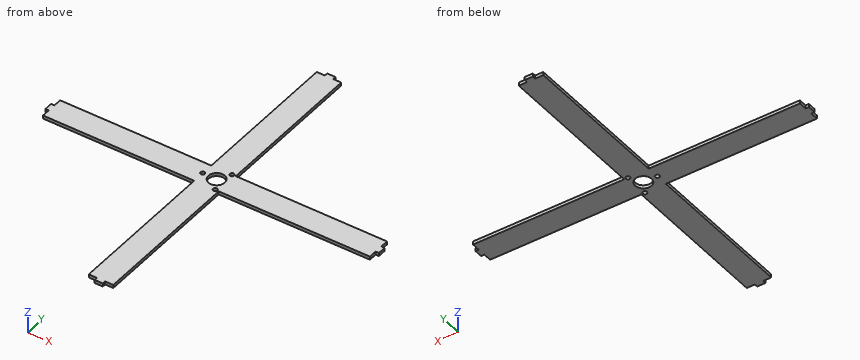
from build123d import *

# Parameters (mm, degrees)
BOSS_EXTRUDE1_DEPTH = 4
CAVITY1_OUTLINE_R   = 2.6
CAVITY1_OUTLINE_R_2 = 10
CAVITY1_DEPTH       = 4


# Read off the part's stored shape, not the designer's step: Cavity1
with BuildPart() as part:
    # Sketch1 → Boss-Extrude1 (new body)
    with BuildSketch(Plane.XY):
        Polygon((363.586470787, 3.889663418), (367.586470787, 3.889663418), (367.586470787, 13.889663418), (363.586470787, 13.889663418), (363.586470787, 23.889663418), (178.577070849, 23.889663418), (178.577070849, 208.900229456), (168.577070849, 208.900229456), (168.577070849, 212.900229456), (158.577070849, 212.900229456), (158.577070849, 208.900229456), (148.577070849, 208.900229456), (148.577070849, 23.889663418), (-36.413529213, 23.889663418), (-36.413529213, 13.889663418), (-40.413529213, 13.889663418), (-40.413529213, 3.889663418), (-36.413529213, 3.889663418), (-36.413529213, -6.110336582), (148.577070849, -6.110336582), (148.577070849, -191.099770544), (158.577070849, -191.099770544), (158.577070849, -195.099770544), (168.577070849, -195.099770544), (168.577070849, -191.099770544), (178.577070849, -191.099770544), (178.577070849, -6.110336582), (363.586470787, -6.110336582), align=None)
    extrude(amount=BOSS_EXTRUDE1_DEPTH)

    # Cavity1 outline → Cavity1 (cut)
    with BuildSketch(Plane.XY):
        with Locations((174.136470787, 23.709263861)):
            Circle(CAVITY1_OUTLINE_R)
        with Locations((174.136470787, -5.908804949)):
            Circle(CAVITY1_OUTLINE_R)
        with Locations((148.486470787, 8.900229456)):
            Circle(CAVITY1_OUTLINE_R)
        with Locations((165.586470787, 8.900229456)):
            Circle(CAVITY1_OUTLINE_R_2)
    extrude(amount=CAVITY1_DEPTH, mode=Mode.SUBTRACT)


solid = part.part
CAD build for the part. Positions are in the model's coordinates, mm. Round coordinates to 2 decimals unless told otherwise and drop trailing zeros. Write each loop counter-clockwise with the first axis right and the second up, starting at its lowest first coordinate (ties: lowest second). Pieces come first, ordered by that corner, then holes. Notation, with made-up numbers: M -34,-34.5 L 10,-34.5 A34 ccw 10,0.5 Z; hole C 64.5,-11.75 d2. An arc over 180 degrees is marked long. Use a Markdown table: item, result. Add a question column.
1. Flat gauge pins, fed straight in: P1, Ø4.5, axis at x = 174.14, y = 23.71, coming from the -Z side; P2, Ø1, axis at y = -5.5, z = 2, coming from the +X side; P3, Ø1, axis at x = 13.5, z = 3, coming from the +Y side; P4, Ø7, axis at x = 148.49, y = 8.9, coming from the +Z side. Where does each tip first touch, or does it go through?
2. Slice it at B-B on x = 185. Give the cut face in (y, z).
3. Slice it at A-A on z = 2.15. Give the number of separate pieces and of enclosed holes in the cut face, then the cut area to 3 significant figures.
4. Drill centre lines: probe 1 along Y at (x, z) = (208, 1.9); probe 2 along Y at (x, z) = (162, 0.4); probe 3 along X at (y, z) = (157, 2.2). Where is each one in solid material? Low to high.
5. Slice it at C-C on y = 155. Give the cut face in (x, z), then the cut area to 3 significant figures.
Reply:
| question | item | result |
|---|---|---|
| 1 | P1 | passes through |
| 1 | P2 | stops at x = 363.59 |
| 1 | P3 | stops at y = 23.89 |
| 1 | P4 | stops at z = 4 |
| 2 | outline | M -6.11,0 L 23.89,0 L 23.89,4 L -6.11,4 Z |
| 3 | separate pieces | 1 |
| 3 | enclosed holes | 4 |
| 3 | area | 22,900 mm^2 |
| 4 | probe 1 | y = -6.11 to 23.89 |
| 4 | probe 2 | y = -195.1 to -0.43, 18.23 to 212.9 |
| 4 | probe 3 | x = 148.58 to 178.58 |
| 5 | outline | M 148.58,0 L 178.58,0 L 178.58,4 L 148.58,4 Z |
| 5 | area | 120 mm^2 |
